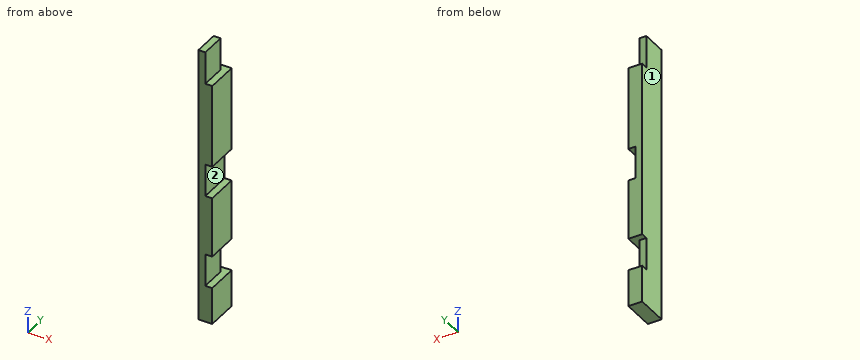
```python
from build123d import *

# Parameters (mm, degrees)
F0_W      = 38.1
F0_H      = 88.9
F1_DEPTH  = 762
F2_W      = 19.05
F2_H      = 88.9
F3_DEPTH  = 88.901
F4_W      = 19.05
F4_H      = 88.9
F5_DEPTH  = 88.901
F6_W      = 19.05
F6_H      = 88.9
F7_DEPTH  = 88.901
F8_W      = 19.05
F8_H      = 88.9
F9_DEPTH  = 19.051
F10_W     = 19.05
F10_H     = 88.9
F11_DEPTH = 19.051


with BuildPart() as f1:
    # F0 (on Top) → F1 (new body)
    with BuildSketch(Plane.XY):
        with Locations((19.05, 44.45)):
            Rectangle(F0_W, F0_H)
    extrude(amount=F1_DEPTH)

    # F2 (on face) → F3 (cut, through all)
    with BuildSketch(Plane.XZ):
        with Locations((28.575, 717.55)):
            Rectangle(F2_W, F2_H)
    extrude(amount=-F3_DEPTH, mode=Mode.SUBTRACT)

    # F4 (on face) → F5 (cut, through all)
    with BuildSketch(Plane.XZ):
        with Locations((28.575, 146.05)):
            Rectangle(F4_W, F4_H)
    extrude(amount=-F5_DEPTH, mode=Mode.SUBTRACT)

    # F6 (on face) → F7 (cut, through all)
    with BuildSketch(Plane.XZ):
        with Locations((28.575, 400.05)):
            Rectangle(F6_W, F6_H)
    extrude(amount=-F7_DEPTH, mode=Mode.SUBTRACT)

    # F8 (on face) → F9 (cut, through all)
    with BuildSketch(Plane.YZ.offset(19.05)):
        with Locations((79.375, 717.55)):
            Rectangle(F8_W, F8_H)
    extrude(amount=-F9_DEPTH, mode=Mode.SUBTRACT)

    # F10 (on face) → F11 (cut, through all)
    with BuildSketch(Plane.YZ.offset(19.05)):
        with Locations((79.375, 146.05)):
            Rectangle(F10_W, F10_H)
    extrude(amount=-F11_DEPTH, mode=Mode.SUBTRACT)


solid = f1.part
```
For this review, take the finished solid that the model builds, in its own axes (mm). Face numbers are marked on the shaded views. Give positions to 0.01 mm unless a question says otherwise; leave off trailing zeros. Write each loop counter-clockwise with the first axis right and the second up, starting at its lowest first coordinate (ties: lowest second). Pieces come first, ordered by that corner, then holes. Notation, with made-up numbers: M -1.5,83.5 L 16.5,83.5 A5 ccw 16.5,92.5 Z; hole C 24,81.25 d1. An arc over 180 degrees is marked long. One line per item, written item: value.
1) Take a section at A-A, the plane x = 29. Write out the cut boundary in (y, z), then the cut area to 3 significant figures.
Results are:
outline: M 0,0 L 88.9,0 L 88.9,101.6 L 0,101.6 Z; M 0,190.5 L 88.9,190.5 L 88.9,355.6 L 0,355.6 Z; M 0,444.5 L 88.9,444.5 L 88.9,673.1 L 0,673.1 Z
area: 44,000 mm²
2) Take a section at D-D, the plane z = 362.5. Write out the cut boundary in (x, y), then the cut area to 3 significant figures.
Results are:
outline: M 0,0 L 19.05,0 L 19.05,88.9 L 0,88.9 Z
area: 1,690 mm²
3) For line 1 (Z direction, x = 31, y = 60.5); line 2 (Z direction, x = 8, y = 79); line 3 (X direction, y = 58.5, z = 431), list the stretches that pass through material, from the lowest coordinate up. Write a range as from..to.
Results are:
line 1: z = 0..101.6, 190.5..355.6, 444.5..673.1
line 2: z = 0..101.6, 190.5..673.1
line 3: x = 0..19.05
4) Take a section at B-B, the plane y = 80. Write out the cut boundary in (x, z).
Results are:
outline: M 0,0 L 38.1,0 L 38.1,101.6 L 0,101.6 Z; M 0,190.5 L 38.1,190.5 L 38.1,355.6 L 19.05,355.6 L 19.05,444.5 L 38.1,444.5 L 38.1,673.1 L 0,673.1 Z
5) The part is to be moulded in two halves that separate along Z. For the marked faces 1 and 2, say which applies: +Z half, -Z half, draft (parallel to the pull), parting line (faces both ways), or undercut.
Results are:
face 1: draft
face 2: undercut
6) Take a section at C-C, the plane y = 9. Write out the cut boundary in (x, z), then the cut area to 3 significant figures.
Results are:
outline: M 0,0 L 38.1,0 L 38.1,101.6 L 19.05,101.6 L 19.05,190.5 L 38.1,190.5 L 38.1,355.6 L 19.05,355.6 L 19.05,444.5 L 38.1,444.5 L 38.1,673.1 L 19.05,673.1 L 19.05,762 L 0,762 Z
area: 24,000 mm²
7) For P1, Ø12, axis at x = 17, z = 175.5, coming from the +Y side; P2, Ø8, axis at x = 29, y = 31.5, coming from the -Z side; P3, Ø1, axis at x = 33.5, y = 66.5, coming from the +Z side, all flat-tipped, find the tip position at first contact; note any pin that passes through.
Results are:
P1: stops at y = 69.85
P2: stops at z = 0
P3: stops at z = 673.1
